For this review, take the finished solid that the model builds, in its own axes (mm). A direction names the side the tool comes from. Coordinates: 2 decimals unless noted, no trailing zeros. Write each loop counter-clockwise with the first axis right and the second up, starting at its lowest first coordinate (ties: lowest second). Pieces come first, ordered by that corner, then holes.
1) Mouldability with a two-part tool opening along Y and no side actions: class faces 1 (the face through (0, 0, 0)), 2 (the face through (23.872, -23.951, 0.254)), 3 (the face through (6.664, 10.416, 0.246)) as pulls with the +Y half, pulls with the -Y half, needs draft (parallel to the pull), parting line crosses it, or undercut.
2) We need section C-C on x = 13.5. Write out the cut boundary in (y, z).
3) We need section B-B on y = 6. Write out the cut boundary in (x, z).
4) To check wall thickness, follow line 1 along Y through (x, z) = (9, 0.3); line 2 along X through (y, z) = (9.5, 0.45); line 3 along Y through (x, z) = (1, 0.2). State the ranges of each line that lie inside material, in increasing order.
5) We need section A-A on z = 0.4. Give the number of separate pieces and of enclosed holes in the cut face, then the cut area to 3 significant figures.
6) For faces 4 (the face through (-18.333, 12.375, 0.254)), 5 (the face through (-23.951, 23.872, 0.254)), list the 3-axis set-ups (+Z, -Z, +X, -X, +Y, -Y) from which the entire face can be reached by the end or side of a thin tool; tool diameter is ignored.
from build123d import *

# Parameters (mm, degrees)
F0_W     = 50.8
F0_H     = 50.8
F1_DEPTH = 0.5
F2_R     = 1.27
F3_R     = 5.08


with BuildPart() as f1:
    # F0 (on Top) → F1 (new body)
    with BuildSketch(Plane.XY):
        Rectangle(F0_W, F0_H)
        Polygon((0, -2.54), (13.97, -19.05), (-13.97, -19.05), align=None, mode=Mode.SUBTRACT)
        Polygon((-19.05, 13.97), (-2.54, 0), (-19.05, -13.97), align=None, mode=Mode.SUBTRACT)
        Polygon((19.05, -13.97), (2.54, 0), (19.05, 13.97), align=None, mode=Mode.SUBTRACT)
        Polygon((13.97, 19.05), (0, 2.54), (-13.97, 19.05), align=None, mode=Mode.SUBTRACT)
    extrude(amount=F1_DEPTH)

    # F2
    f2_edges = [f1.edges().sort_by_distance(p)[0] for p in [
        (0, -2.54, 0.25),
        (-19.05, 13.97, 0.25),
        (-13.97, -19.05, 0.25),
        (2.54, 0, 0.25),
        (19.05, -13.97, 0.25),
        (13.97, -19.05, 0.25),
        (-2.54, 0, 0.25),
        (0, 2.54, 0.25),
        (19.05, 13.97, 0.25),
        (13.97, 19.05, 0.25),
        (-19.05, -13.97, 0.25),
        (-13.97, 19.05, 0.25),
    ]]
    fillet(f2_edges, radius=F2_R)

    # F3
    f3_edges = [f1.edges().sort_by_distance(p)[0] for p in [
        (25.4, 25.4, 0.25),
        (-25.4, 25.4, 0.25),
        (-25.4, -25.4, 0.25),
        (25.4, -25.4, 0.25),
    ]]
    fillet(f3_edges, radius=F3_R)


solid = f1.part
Result:
1. face 1: needs draft
1. face 2: pulls with the -Y half
1. face 3: undercut
2. outline: (-25.4, 0) - (-9.27, 0) - (-9.27, 0.5) - (-25.4, 0.5) - close; (9.27, 0) - (25.4, 0) - (25.4, 0.5) - (9.27, 0.5) - close
3. outline: (-25.4, 0) - (-19.05, 0) - (-19.05, 0.5) - (-25.4, 0.5) - close; (-9.63, 0) - (-2.93, 0) - (-2.93, 0.5) - (-9.63, 0.5) - close; (2.93, 0) - (9.63, 0) - (9.63, 0.5) - (2.93, 0.5) - close; (19.05, 0) - (25.4, 0) - (25.4, 0.5) - (19.05, 0.5) - close
4. line 1: y = -25.4 to -19.05, -13.18 to -5.47, 5.47 to 13.18, 19.05 to 25.4
4. line 2: x = -25.4 to -19.05, -13.77 to -5.89, 5.89 to 13.77, 19.05 to 25.4
4. line 3: y = -25.4 to -19.05, -3.72 to 3.72, 19.05 to 25.4
5. separate pieces: 1
5. enclosed holes: 4
5. area: 1,650 mm2
6. face 4: +Z, -Z
6. face 5: +Z, -Z, -X, +Y
